Answer from the drawing. Dimensions are ordinates in mm from the lowest x, y and z of the part. A direction names the side the tool comes from. Coordinates: 2 decimals unless noted, no trailing zeros. Write each loop counter-clockwise with the first axis right and the second up, starting at its lowest first coordinate (ties: lowest second). Pieces come first, ordered by that corner, then holes. Notation, with made-up numbers: M 21.5,78.5 L 47.5,78.5 A14 ccw 47.5,84.5 Z; hole C 18,79 d11. An arc over 180 degrees is marked long. Put each result on its own line as item: value. Start each with the question number.
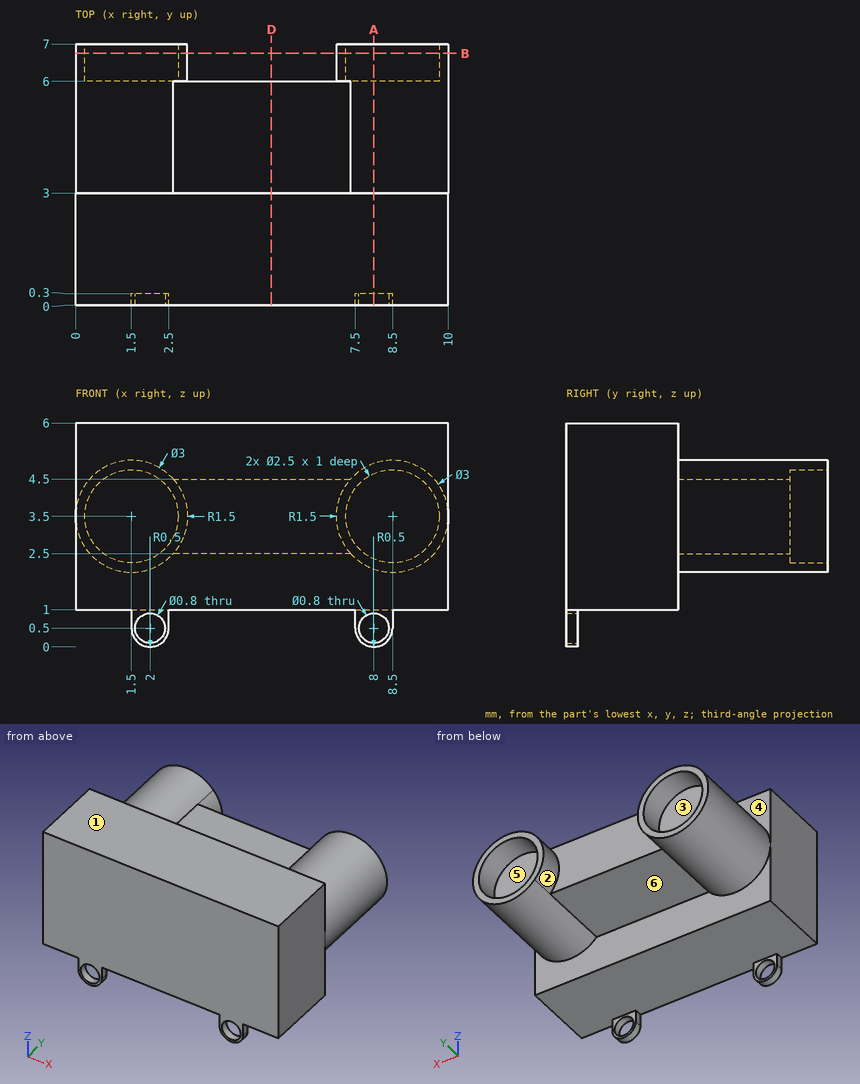
1) Straight lines are drawn through the part: probe 1 along Y at (x, z) = (5.5, 5.05); probe 2 along Z at (x, y) = (5.75, 1); probe 3 along Y at (x, z) = (5.75, 4.45). For each, find the intervals that lie inside material, in ascending order.
2) Given pin 1 Ø2.5 at (x, y) = (4.5, 5) entering from +Z; pin 2 Ø1.5 at (x, y) = (4, 5) entering from -Z; pin 3 Ø2 at (x, z) = (8.5, 3.5) entering from +Y, each flat-ended and moving along its own axis, determine where each tip first touches the part or whether it passes through.
3) Determine the mould class of the marked faces 1, 2 and 3 for opening direction Z: +Z half, -Z half, draft (parallel to the pull), parting line (faces both ways), or undercut.
4) A cutting plane is placed at A-A on x = 8. Write down the section's boundary in (y, z).
5) A cutting plane is placed at D-D on x = 5.25. Write down the section's boundary in (y, z).
6) A cutting plane is placed at B-B on y = 6.75. Write down the section's boundary in (x, z), then the cut area to 3 significant figures.
7) For the marked faces 4, 5 and 6, determine the directions among +Z, -Z, +X, -X, +Y, -Y from which every point of the face is accessible in a straight line to the end or side of a thin tool.
Answers follow:
1. probe 1: y = 0 to 3
1. probe 2: z = 1 to 6
1. probe 3: y = 0 to 6
2. pin 1: stops at z = 4.5
2. pin 2: stops at z = 2.5
2. pin 3: stops at y = 6
3. face 1: +Z half
3. face 2: parting line
3. face 3: undercut
4. outline: M 0,0 L 0.3,0 L 0.3,0.1 L 0,0.1 Z; M 0,0.9 L 0.3,0.9 L 0.3,1 L 3,1 L 3,2.09 L 7,2.09 L 7,2.35 L 6,2.35 L 6,4.65 L 7,4.65 L 7,4.91 L 3,4.91 L 3,6 L 0,6 Z
5. outline: M 0,1 L 3,1 L 3,2.5 L 6,2.5 L 6,4.5 L 3,4.5 L 3,6 L 0,6 Z
6. outline: C 1.5,3.5 d3; C 8.5,3.5 d3; hole C 1.5,3.5 d2.5; hole C 8.5,3.5 d2.5
6. area: 4.32 mm²
7. face 4: +Z, +Y
7. face 5: +Y
7. face 6: -Z, +Y
